```python
from build123d import *

# Parameters (mm, degrees)
SKETCH1_W           = 56
SKETCH1_H           = 60
SKETCH1_W_2         = 50
SKETCH1_H_2         = 54
BOSS_EXTRUDE1_DEPTH = 24
SKETCH2_W           = 56
SKETCH2_H           = 60
BOSS_EXTRUDE2_DEPTH = 3
CUT_EXTRUDE1_DEPTH  = 12.5
BOSS_EXTRUDE3_DEPTH = 12
SKETCH5_W           = 53.4
SKETCH5_H           = 57.4
SKETCH5_W_2         = 50
SKETCH5_H_2         = 54
CUT_EXTRUDE2_DEPTH  = 5.5
CUT_EXTRUDE3_REACH  = 58.267
SKETCH6_W           = 6
SKETCH6_H           = 12
FILLET3_R           = 3


with BuildPart() as part:
    # Sketch1 → Boss-Extrude1 (new body)
    with BuildSketch(Plane(origin=(0, 9.820251789, 0), x_dir=(1, 0, 0), z_dir=(0, 1, 0))):
        Rectangle(SKETCH1_W, SKETCH1_H)
        Rectangle(SKETCH1_W_2, SKETCH1_H_2, mode=Mode.SUBTRACT)
    extrude(amount=BOSS_EXTRUDE1_DEPTH)

    # Sketch2 → Boss-Extrude2 (add)
    with BuildSketch(Plane(origin=(0, 33.820251789, 0), x_dir=(1, 0, 0), z_dir=(0, 1, 0))):
        Rectangle(SKETCH2_W, SKETCH2_H)
    extrude(amount=BOSS_EXTRUDE2_DEPTH)

    # Sketch3 → Cut-Extrude1 (cut, symmetric)
    with BuildSketch(Plane(origin=(0, 0, 0), x_dir=(0, 0, -1), z_dir=(1, 0, 0))):
        Polygon((28.5, 9.820251789), (28.5, 23.320251789), (30, 24.820251789), (30, 9.820251789), align=None)
    cut_extrude1 = extrude(amount=CUT_EXTRUDE1_DEPTH, both=True, mode=Mode.SUBTRACT)

    # Sketch4 → Boss-Extrude3 (add, symmetric)
    with BuildSketch(Plane(origin=(0, 0, 0), x_dir=(0, 0, -1), z_dir=(1, 0, 0))):
        Polygon((30.1, 7.070251789), (28.5, 7.070251789), (28.5, 6.420251789), (30.5, 4.420251789), (32.5, 6.420251789), (36.5, 4.420251789), (36.5, 9.420251789), (31, 16.420251789), (31, 35.820251789), (30, 36.820251789), (29, 36.820251789), (29, 10.734465351), (30.1, 9.634465351), align=None)
    boss_extrude3 = extrude(amount=BOSS_EXTRUDE3_DEPTH, both=True)

    # Sketch5 → Cut-Extrude2 (cut)
    with BuildSketch(Plane.XZ.offset(-9.820251789)):
        Rectangle(SKETCH5_W, SKETCH5_H)
        Rectangle(SKETCH5_W_2, SKETCH5_H_2, mode=Mode.SUBTRACT)
    extrude(amount=-CUT_EXTRUDE2_DEPTH, mode=Mode.SUBTRACT)

    # Mirror1: Cut-Extrude1, Boss-Extrude3 across plane
    add(cut_extrude1.mirror(Plane.XY), mode=Mode.SUBTRACT)
    add(boss_extrude3.mirror(Plane.XY))

    # Sketch6 → Cut-Extrude3 (cut, up to next)
    with BuildSketch(Plane(origin=(0, 36.820251789, 0), x_dir=(1, 0, 0), z_dir=(0, 1, 0)), mode=Mode.PRIVATE) as cut_extrude3_sk1:
        with Locations((5, 0)):
            Rectangle(SKETCH6_W, SKETCH6_H)
    cut_extrude3_tool1 = extrude(cut_extrude3_sk1.sketch, amount=-CUT_EXTRUDE3_REACH, mode=Mode.PRIVATE) & part.part
    add(cut_extrude3_tool1.solids().sort_by_distance((5, 36.820252, 0))[0], mode=Mode.SUBTRACT)

    # Fillet3
    fillet3_edges = [part.edges().sort_by_distance(p)[0] for p in [
        (2, 35.320251789, 6),
        (8, 35.320251789, 6),
        (8, 35.320251789, -6),
        (2, 35.320251789, -6),
    ]]
    fillet(fillet3_edges, radius=FILLET3_R - 0.0001)  # a hair under: the kernel refuses the full size


solid = part.part
```
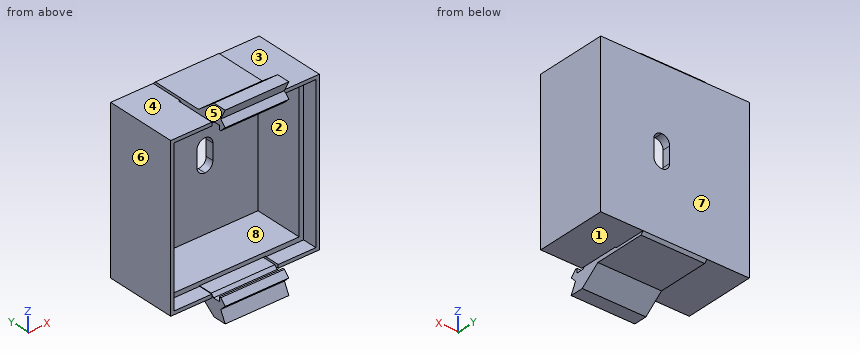
Read the model definition and answer for the solid it produces. Units are mm, in the model's axes. Face numbers are marked on the shaded views. A direction names the side the tool comes from. Coordinates: 2 decimals unless noted, no trailing zeros. Write each loop counter-clockwise with the first axis right and the second up, starting at its lowest first coordinate (ties: lowest second). Pieces come first, ordered by that corner, then holes. Notation, with made-up numbers: (-31.75, 4.5) - (-18.75, 4.5) arc R10 cw to (-18.75, 13.5) - close; hole circle Ø4 at (-37, 78). An arc over 180 degrees is marked (long way). Answer as a JSON object with one key per item and string values. Group by question number.
1. Consider L1, parallel to Z at x = 10, y = 19; L2, parallel to Z at x = -10.5, y = 9; L3, parallel to X at y = 30.5, z = -9. Determine where each line is inside the solid, lowest interval first. Write a range as [from, to].
2. A cutting plane is placed at B-B (z = 0.5). Determine the outline of the cut face in (x, y), plus the area to 3 significant figures.
3. A cutting plane is placed at D-D (x = 23.5). Determine the outline of the cut face in (y, z).
4. A cutting plane is placed at A-A (y = 18). Determine the outline of the cut face in (x, z).
5. A cutting plane is placed at C-C (y = 32). Determine the outline of the cut face in (x, z).
6. The mould has two halves that part along X. Classify the marked faces 5, 6, 7 and 8: +X half, -X half, draft (parallel to the pull), parting line (faces both ways), or undercut.
7. Each of these flat-tipped pins is pushed along its axis until it touches: P1, Ø5, axis at x = 19.5, y = 23.5, coming from the -Z side; P2, Ø5, axis at x = -7, y = 26.5, coming from the +Z side; P3, Ø2, axis at x = -12, z = -4.5, coming from the -Y side; P4, Ø4, axis at y = 23.5, z = 34, coming from the -X side. Where does it stop, or does it pass through?
8. Which of the six approach directions +Z, -Z, +X, -X, +Y, -Y give full straight-line access (tool end or side, diameter ignored) to the marked faces 1, 2, 3 and 4?
Worked out:
{
 "1": {"L1": "z = [-31, -29], [-28.5, -27], [27, 28.5], [29, 31]", "L2": "z = [-36.5, -30.1], [30.1, 36.5]", "L3": "x = [-28, -25], [25, 28]"},
 "2": {"outline": "(-28, 9.82) - (-26.7, 9.82) - (-26.7, 15.32) - (-25, 15.32) - (-25, 33.82) - (2, 33.82) - (2, 36.82) - (-28, 36.82) - close; (8, 33.82) - (25, 33.82) - (25, 15.32) - (26.7, 15.32) - (26.7, 9.82) - (28, 9.82) - (28, 36.82) - (8, 36.82) - close", "area": "275 mm²"},
 "3": {"outline": "(9.82, -30) - (36.82, -30) - (36.82, 30) - (9.82, 30) - (9.82, 28.7) - (15.32, 28.7) - (15.32, 27) - (33.82, 27) - (33.82, -27) - (15.32, -27) - (15.32, -28.7) - (9.82, -28.7) - close"},
 "4": {"outline": "(-28, -30) - (-12.5, -30) - (-12.5, -28.5) - (12.5, -28.5) - (12.5, -30) - (28, -30) - (28, 30) - (12.5, 30) - (12.5, 28.5) - (-12.5, 28.5) - (-12.5, 30) - (-28, 30) - close; (-12, -31) - (12, -31) - (12, -29) - (-12, -29) - close; (-12, 29) - (12, 29) - (12, 31) - (-12, 31) - close; hole (-25, -27) - (25, -27) - (25, 27) - (-25, 27) - close"},
 "5": {"outline": "(-28, -30) - (-12, -30) - (-12, -31) - (12, -31) - (12, -30) - (28, -30) - (28, 30) - (12, 30) - (12, 31) - (-12, 31) - (-12, 30) - (-28, 30) - close; hole (-25, -27) - (25, -27) - (25, 27) - (-25, 27) - close"},
 "6": {"face 5": "undercut", "face 6": "-X half", "face 7": "draft", "face 8": "undercut"},
 "7": {"P1": "stops at z = -30", "P2": "stops at z = 31", "P3": "stops at y = 33.82", "P4": "passes through"},
 "8": {"face 1": "-Z, +X, +Y, -Y", "face 2": "-Y", "face 3": "+Z, +X, +Y, -Y", "face 4": "+Z, -X, +Y, -Y"}
}
